Source: CAD feature listing. Evaluate the final solid. Frame: model axes, mm. Face numbers are marked on the shaded views. Give positions to 0.01 mm unless a question says otherwise; leave off trailing zeros. Order: outer loops, then holes, each group sorted by start corner. A loop starts at its lowest first (then second) coordinate and runs counter-clockwise, first axis right, second up.
1) First-contact query: P1, Ø2, axis at x = 1, y = 0, coming from the +Z side; P2, Ø1.8, axis at x = -0.5, z = -0.5, coming from the +Y side; P3, Ø3, axis at x = 1, z = -23, coming from the +Y side. Flat tips, straight axial feed; report the tip coordinate or a pass-through.
2) Draft query along Y for the marked faces 1, 2, 3 and 4. Return one class per face: released by +Y, released by -Y, zero draft, split by the parting line, or undercut.
3) Material intervals for line 1 (Y direction, x = 0, z = -23.75); line 2 (Z direction, x = 1, y = -0.75); line 3 (Z direction, x = 1.25, y = 2), sorted ascending.
4) Section A-A, the plane z = -14. Return loops of the section in (x, y).
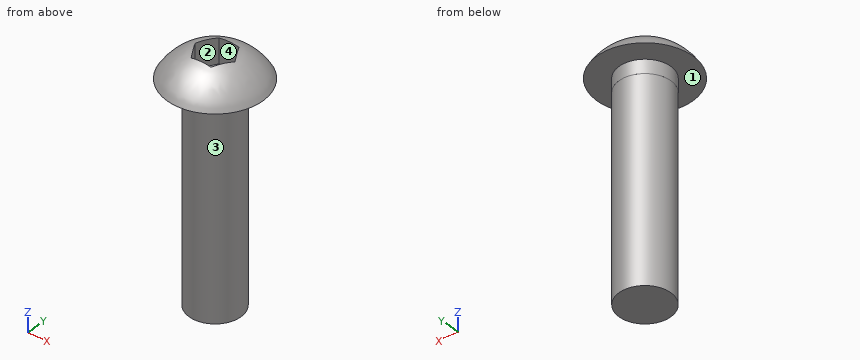
Solid Edge part; units mm, degrees
sketch "Sketch1" plane through (0, 0, 0) normal (1, 0, 0) x (0, 1, 0)
  line L0 (0, -1.6764) -> (0, 1.6764)
  arc A0 (0, 1.6764) -> (5.55625, -1.6764) centre (-0.25374, -5.024398) cw
  line L1 (0, -1.6764) -> (5.55625, -1.6764)
revolve "RevolvedProtrusion1" add sketch "Sketch1" angle 360 about axis through (0, 0, -14.779625) along (0, 0, 1)
sketch "Sketch2" plane through (0, 0, -1.6764) normal (0, 0, -1) x (0, 1, 0)
  circle A0 centre (0, 0) radius 3
extrude "Protrusion1" add sketch "Sketch2" along normal blind 25
sketch "Sketch3" plane through (0, 0, -26.6764) normal (0, 0, -1) x (1, 0, 0)
  circle A0 centre (0, 0) radius 2.99746
extrude "Cutout1" cut sketch "Sketch3" against normal blind 23.4125 flip side to cut
sketch "Sketch4" plane through (-0.603226, 0.360624, 3.3528) normal (0, 0, 1) x (1, 0, 0)
  line L0 (-0.551475, 1.639376) -> (1.757926, 1.639376)
  line L1 (2.912627, -0.360624) -> (1.757926, 1.639376)
  line L2 (1.757926, -2.360624) -> (2.912627, -0.360624)
  line L3 (-0.551475, -2.360624) -> (1.757926, -2.360624)
  line L4 (-1.706175, -0.360624) -> (-0.551475, -2.360624)
  line L5 (-0.551475, 1.639376) -> (-1.706175, -0.360624)
extrude "ExtrudedCutout_11" cut sketch "Sketch4" against normal blind 5.0292
properties part number "185818"
From the geometry:
1. P1: stops at z = -1.68
1. P2: stops at y = 5.37
1. P3: stops at y = 3
2. face 1: zero draft
2. face 2: undercut
2. face 3: split by the parting line
2. face 4: undercut
3. line 1: y = -3 to 3
3. line 2: z = -26.68 to -1.68
3. line 3: z = -26.68 to 1.15
4. outline: circle Ø5.99 at (0, 0)
